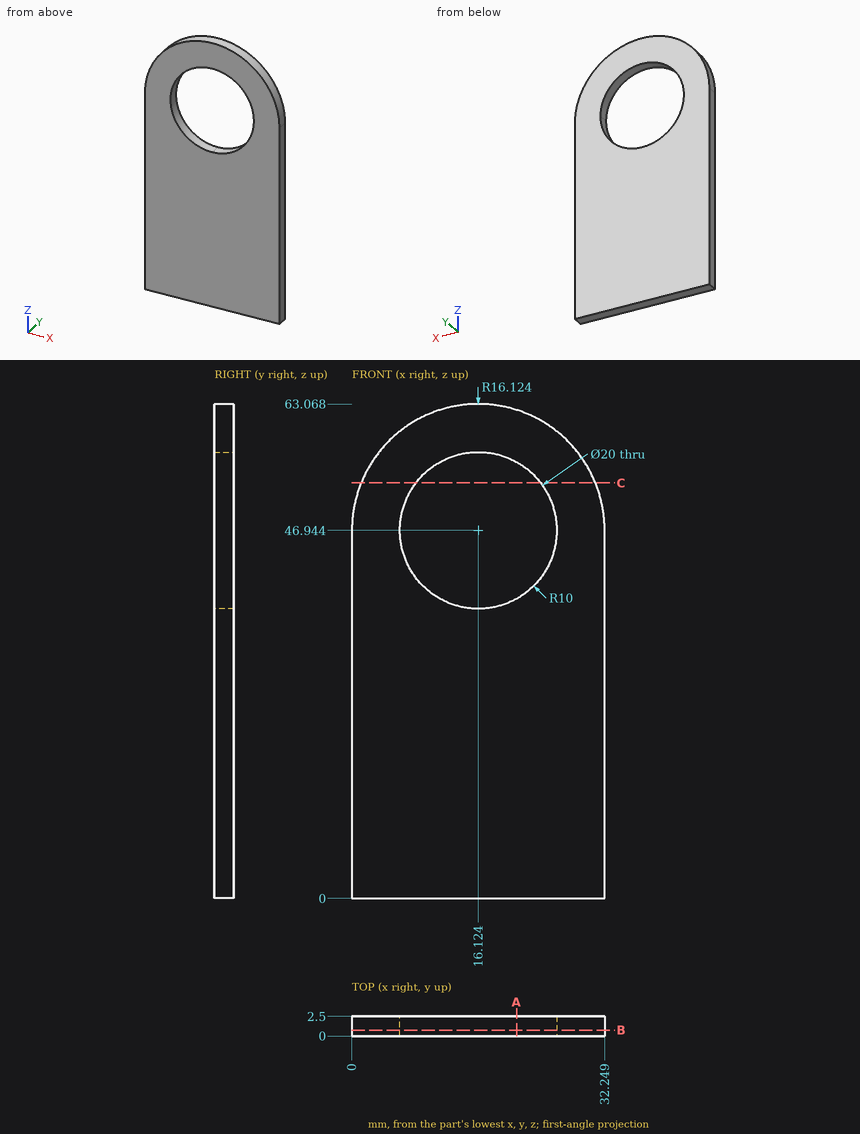
Study the drawing (mm; zero at the part's minimum x, y, z) and answer. Round coordinates to 2 decimals unless told otherwise and drop trailing zeros. Write each loop counter-clockwise with the first axis right and the second up, starting at its lowest first coordinate (ties: lowest second). Pieces come first, ordered by that corner, then holes. Notation, with made-up numbers: (69, -24.5) -> (96, -24.5) arc R25 cw to (96, 4.5) -> close; hole circle Ø11 at (62, 59). An arc over 180 degrees is marked (long way). Use CSV: the item, a comma, the result in double quotes. Start each with the question number.
(1) Section A-A on x = 21 is taken. Give the vertices of the cut face in (y, z) (1 decimal).
(2) Section B-B on y = 0.75 is taken. Give the vertices of the cut face in (x, z) (1 decimal), then the cut area to 3 significant figures.
(3) Consider L1, parallel to Z at x = 9.5, y = 0.9 (1 decimal); L2, parallel to Z at x = 10, y = 1.25; L3, parallel to X at y = 0.95, z = 50 (1 decimal). Determine where each line is inside the solid, lowest interval first. Write a range as from..to.
(4) Section C-C on z = 53 is taken. Give the vertices of the cut face in (x, y).
A:
1,outline,"(0, 0) -> (2.5, 0) -> (2.5, 38.2) -> (0, 38.2) -> close; (0, 55.7) -> (2.5, 55.7) -> (2.5, 62.3) -> (0, 62.3) -> close"
2,outline,"(0, 0) -> (32.2, 0) -> (32.2, 46.9) arc R16.1 ccw to (0, 46.9) -> close; hole circle Ø20 at (16.1, 46.9)"
2,area,"1,610 mm²"
3,L1,"z = 0..39.5, 54.4..61.6"
3,L2,"z = 0..39.04, 54.85..61.86"
3,L3,"x = 0.3..6.6, 25.6..32"
4,outline,"(1.18, 0) -> (8.17, 0) -> (8.17, 2.5) -> (1.18, 2.5) -> close; (24.08, 0) -> (31.07, 0) -> (31.07, 2.5) -> (24.08, 2.5) -> close"
